from build123d import *

# Parameters (mm, degrees)
EXTRUDE_1_DEPTH                 = 20.5
CUT_EXTRUDE_1_REACH             = 27.889
CUT_EXTRUDE_1_DIRECTION_2_REACH = 27.889


with BuildPart() as part:
    # Эскиз1 → Бобышка-Вытянуть1 (new, symmetric)
    with BuildSketch(Plane(origin=(0, 0, 0), x_dir=(1, 0, 0), z_dir=(0, 1, 0))):
        with BuildLine():
            Line((-14, 0), (14, 0))
            ThreePointArc((14, 0), (14.707106781, -0.292893219), (15, -1))
            Line((15, -1), (15, -2.7))
            ThreePointArc((15, -2.7), (14.7, -3), (14.4, -2.7))
            Line((14.4, -2.7), (14.4, -1.1))
            ThreePointArc((14.4, -1.1), (14.3, -1), (14.2, -1.1))
            Line((14.2, -1.1), (14.2, -3))
            ThreePointArc((14.2, -3), (13.614213562, -4.414213562), (12.2, -5))
            Line((12.2, -5), (-12.2, -5))
            ThreePointArc((-12.2, -5), (-13.614213562, -4.414213562), (-14.2, -3))
            Line((-14.2, -3), (-14.2, -1.1))
            ThreePointArc((-14.2, -1.1), (-14.3, -1), (-14.4, -1.1))
            Line((-14.4, -1.1), (-14.4, -2.7))
            ThreePointArc((-14.4, -2.7), (-14.7, -3), (-15, -2.7))
            Line((-15, -2.7), (-15, -1))
            ThreePointArc((-15, -1), (-14.707106781, -0.292893219), (-14, 0))
        make_face()
    extrude(amount=EXTRUDE_1_DEPTH, both=True)

    # Эскиз2 → Вырез-Вытянуть1 (cut, up to next)
    with BuildSketch(Plane(origin=(0, 0, 0), x_dir=(0, 0, -1), z_dir=(1, 0, 0)), mode=Mode.PRIVATE) as cut_extrude_1_sk1:
        with BuildLine():
            Line((-3, 19.85), (-3, 14.65))
            ThreePointArc((-3, 14.65), (-3.190380592, 14.190380592), (-3.65, 14))
            Line((-3.65, 14), (-4.35, 14))
            ThreePointArc((-4.35, 14), (-4.809619408, 13.809619408), (-5, 13.35))
            Line((-5, 13.35), (-5, 20.5))
            Line((-5, 20.5), (-2.35, 20.5))
            ThreePointArc((-2.35, 20.5), (-2.809619408, 20.309619408), (-3, 19.85))
        make_face()
    cut_extrude_1_tool1 = extrude(cut_extrude_1_sk1.sketch, amount=-CUT_EXTRUDE_1_REACH, mode=Mode.PRIVATE) & part.part
    add(cut_extrude_1_tool1.solids().sort_by_distance((0, 17.269493, 4.003909))[0], mode=Mode.SUBTRACT)

    # Эскиз2 → Вырез-Вытянуть1 direction 2 (cut, up to next)
    with BuildSketch(Plane(origin=(0, 0, 0), x_dir=(0, 0, -1), z_dir=(1, 0, 0)), mode=Mode.PRIVATE) as cut_extrude_1_direction_2_sk1:
        with BuildLine():
            Line((-3, 19.85), (-3, 14.65))
            ThreePointArc((-3, 14.65), (-3.190380592, 14.190380592), (-3.65, 14))
            Line((-3.65, 14), (-4.35, 14))
            ThreePointArc((-4.35, 14), (-4.809619408, 13.809619408), (-5, 13.35))
            Line((-5, 13.35), (-5, 20.5))
            Line((-5, 20.5), (-2.35, 20.5))
            ThreePointArc((-2.35, 20.5), (-2.809619408, 20.309619408), (-3, 19.85))
        make_face()
    cut_extrude_1_direction_2_tool1 = extrude(cut_extrude_1_direction_2_sk1.sketch, amount=CUT_EXTRUDE_1_DIRECTION_2_REACH, mode=Mode.PRIVATE) & part.part
    add(cut_extrude_1_direction_2_tool1.solids().sort_by_distance((0, 17.269493, 4.003909))[0], mode=Mode.SUBTRACT)


solid = part.part
Check sheet for the modelled part. Datum: model origin and axes. Units: mm. A direction names the side the tool comes from. Round coordinates to 2 decimals unless told otherwise and drop trailing zeros. Loops run counter-clockwise (first coordinate to the right, second up) from the corner with the lowest first, then second, coordinate; pieces in that order, holes last.
1. Mould release check, pull along X, two halves, no side actions. Record for faces 4 (the flat face through (14.2, 0, 2)), 5 (the flat face through (0, -3, 5)), 6 (the flat face through (-15, 0, 2)): released by +X, released by -X, zero draft, split by the parting line, or undercut.
2. Set-up check for faces 1 (the flat face through (0, 17, 3)), 2 (the flat face through (0, 0, 0)), 3 (the flat face through (-14.2, 0, 2)): record each of +Z, -Z, +X, -X, +Y, -Y from which the full face is reachable in a straight line by a thin tool's end or side.
3. Scan lines: probe 1 along X at (y, z) = (14.5, 2.7); probe 2 along Y at (x, z) = (-11.75, 4); probe 3 along X at (y, z) = (-5, 2.95). Record each from-to range of solid material in increasing order.
4. Sectioned sample at B-B on y = 4. Record the boundary of the cut face in (x, z).
5. Sectioned sample at A-A on x = 4.5. Record the boundary of the cut face in (y, z), and give its area (3 significant figures).
6. Sectioned sample at C-C on y = 17. Record the boundary of the cut face in (x, z).
7. Gauge pin test, flat end, axial feed: pin 1 Ø5.5 at (x, y) = (4, 18) entering from +Z. Record the tip position at first contact, or that the pin passes through.
Recorded:
1. face 4: undercut
1. face 5: zero draft
1. face 6: released by -X
2. face 1: +Z, +X, -X, +Y
2. face 2: -Z, +X, -X, +Y, -Y
2. face 3: +Z, +Y, -Y
3. probe 1: x = -15 to -14.4, -14.2 to 14.2, 14.4 to 15
3. probe 2: y = -20.5 to 14
3. probe 3: x = -14.87 to -14.53, -14.2 to 14.2, 14.53 to 14.87
4. outline: (-15, 1) arc R1 ccw to (-14, 0) - (14, 0) arc R1 ccw to (15, 1) - (15, 2.7) arc R0.3 ccw to (14.4, 2.7) - (14.4, 1.1) arc R0.1 cw to (14.2, 1.1) - (14.2, 3) arc R2 ccw to (12.2, 5) - (-12.2, 5) arc R2 ccw to (-14.2, 3) - (-14.2, 1.1) arc R0.1 cw to (-14.4, 1.1) - (-14.4, 2.7) arc R0.3 ccw to (-15, 2.7) - close
5. outline: (-20.5, 0) - (20.5, 0) - (20.5, 2.35) arc R0.65 ccw to (19.85, 3) - (14.65, 3) arc R0.65 cw to (14, 3.65) - (14, 4.35) arc R0.65 ccw to (13.35, 5) - (-20.5, 5) - close
5. area: 192 mm2
6. outline: (-15, 1) arc R1 ccw to (-14, 0) - (14, 0) arc R1 ccw to (15, 1) - (15, 2.7) arc R0.3 ccw to (14.4, 2.7) - (14.4, 1.1) arc R0.1 cw to (14.2, 1.1) - (14.2, 3) - (-14.2, 3) - (-14.2, 1.1) arc R0.1 cw to (-14.4, 1.1) - (-14.4, 2.7) arc R0.3 ccw to (-15, 2.7) - close
7. pin 1: stops at z = 3
